Check sheet for the modelled part. Datum: model origin and axes. Units: mm. Round coordinates to 2 decimals unless told otherwise and drop trailing zeros. Write each loop counter-clockwise with the first axis right and the second up, starting at its lowest first coordinate (ties: lowest second). Pieces come first, ordered by that corner, then holes. Notation, with made-up numbers: (60, 74.5) -> (77, 74.5) arc R18 ccw to (77, 79.5) -> close; hole circle Ø4 at (-0.75, 41). An arc over 180 degrees is marked (long way). Answer as a JSON object with one key per item and string values. Group by question number.
```python
from build123d import *

# Parameters (mm, degrees)
BOSS_EXTRUDE12_DEPTH       = 1
SKETCH88_W                 = 60
SKETCH88_H                 = 110
CUT_EXTRUDE1_DEPTH         = 1
FILLET1_R                  = 10
M2_5_CLEARANCE_HOLE1_D     = 2.9
M2_5_CLEARANCE_HOLE1_DEPTH = 11.5
SKETCH91_W                 = 8
SKETCH91_H                 = 15
SKETCH91_R                 = 1.55
BOSS_EXTRUDE13_DEPTH       = 1
FILLET2_R                  = 2
CHAMFER1_SIZE              = 1.5
SKETCH93_R                 = 1.25
CUT_EXTRUDE2_DEPTH         = 10
M2_5_CLEARANCE_HOLE2_D     = 2.9
M2_5_CLEARANCE_HOLE2_DEPTH = 30


with BuildPart() as part:
    # Sketch87 → Boss-Extrude12 (new body)
    with BuildSketch(Plane.XY):
        Polygon((-40, 70), (-40, -70), (-30, -70), (-30, -60), (30, -60), (30, -70), (40, -70), (40, 70), align=None)
    extrude(amount=BOSS_EXTRUDE12_DEPTH)

    # Sketch88 → Cut-Extrude1 (cut)
    with BuildSketch(Plane.XY.offset(1)):
        with Locations((0, 5)):
            Rectangle(SKETCH88_W, SKETCH88_H)
    extrude(amount=-CUT_EXTRUDE1_DEPTH, mode=Mode.SUBTRACT)

    # Fillet1
    fillet1_edges = [part.edges().sort_by_distance(p)[0] for p in [
        (-30, -50, 0.5),
        (-30, 60, 0.5),
        (30, 60, 0.5),
        (30, -50, 0.5),
    ]]
    fillet(fillet1_edges, radius=FILLET1_R)

    # M2.5 Clearance Hole1
    with Locations(Plane(origin=(0, 0, 0), x_dir=(-1, 0, 0), z_dir=(0, 0, -1))):
        with Locations((35, -65), (35, -55), (-35, -55), (-35, -65), (12, -55), (-12, -55), (-12, 65), (12, 65), (-35, 65), (35, 65), (-35, 55), (35, 55)):
            Hole(M2_5_CLEARANCE_HOLE1_D / 2, depth=M2_5_CLEARANCE_HOLE1_DEPTH)

    # Sketch91 → Boss-Extrude13 (add)
    with BuildSketch(Plane(origin=(0, 0, 0), x_dir=(-1, 0, 0), z_dir=(0, 0, -1))):
        with Locations((-9, -67.5)):
            Rectangle(SKETCH91_W, SKETCH91_H)
        with Locations((-9, -70.5)):
            Circle(SKETCH91_R, mode=Mode.SUBTRACT)
    extrude(amount=-BOSS_EXTRUDE13_DEPTH)

    # Fillet2
    fillet2_edges = [part.edges().sort_by_distance(p)[0] for p in [
        (30, -60, 0.5),
        (-30, -60, 0.5),
        (13, -60, 0.5),
    ]]
    fillet(fillet2_edges, radius=FILLET2_R)

    # Chamfer1
    chamfer1_edges = [part.edges().sort_by_distance(p)[0] for p in [
        (40, 70, 0.5),
        (40, -70, 0.5),
        (-40, -70, 0.5),
        (-40, 70, 0.5),
    ]]
    chamfer(chamfer1_edges, length=CHAMFER1_SIZE)

    # Sketch93 → Cut-Extrude2 (cut)
    with BuildSketch(Plane(origin=(0, 0, 0), x_dir=(-1, 0, 0), z_dir=(0, 0, -1))):
        with Locations((-4.292893219, -60.707106781)):
            Circle(SKETCH93_R)
    extrude(amount=-CUT_EXTRUDE2_DEPTH, mode=Mode.SUBTRACT)

    # M2.5 Clearance Hole2
    with Locations(Plane(origin=(0, 0, 0), x_dir=(-1, 0, 0), z_dir=(0, 0, -1))):
        with Locations((-36, 14), (-36, -6)):
            m2_5_clearance_hole2 = Hole(M2_5_CLEARANCE_HOLE2_D / 2, depth=M2_5_CLEARANCE_HOLE2_DEPTH)

    # Mirror1: M2.5 Clearance Hole2 across plane
    add(m2_5_clearance_hole2.mirror(Plane(origin=(0, 0, 0), x_dir=(0, 0, 1), z_dir=(1, 0, 0))), mode=Mode.SUBTRACT)


solid = part.part
```
(1) Scan lines: line 1 along Y through (x, z) = (9, 0.3); line 2 along X through (y, z) = (-65, 0.35); line 3 along X through (y, z) = (65, 0.65). Record each from-to range of solid material in increasing order.
(2) Section check C-C on x = -12. Record the cut outline in (y, z), then the cut area to 3 significant figures.
(3) Go/stop test with flat-tipped pins: pin 1 Ø2.5 at (x, y) = (-12, -55) entering from +Z; pin 2 Ø3.5 at (x, y) = (12, 65) entering from -Z. Record where each tip stops, or that it passes through.
(4) Section check A-A on x = 9. Record the cut outline in (y, z), then the cut area to 3 significant figures.
(5) Section check D-D on x = -23.5. Record the cut outline in (y, z), then the cut area to 3 significant figures.
(6) Release check for a two-part mould opening along Y. For faces 1 (the flat face through (-33, 3, 0)), 2 (the cylindrical face through (-34.85, -6.88, 0.51)), 3 (the cylindrical face through (-26.99, -47.15, 0.49)) record: pulls with the +Y half, pulls with the -Y half, needs draft (parallel to the pull), parting line crosses it, or undercut.
(7) Section check B-B on y = -11. Record the cut outline in (x, z).
Data:
{
 "1": {"line 1": "y = -75 to -72.05, -68.95 to -50, 60 to 70", "line 2": "x = -40 to -36.45, -33.55 to -30, 5 to 13, 30 to 33.55, 36.45 to 40", "line 3": "x = -40 to -36.45, -33.55 to -13.45, -10.55 to 10.55, 13.45 to 33.55, 36.45 to 40"},
 "2": {"outline": "(-60, 0) -> (-56.45, 0) -> (-56.45, 1) -> (-60, 1) -> close; (-53.55, 0) -> (-50, 0) -> (-50, 1) -> (-53.55, 1) -> close; (60, 0) -> (63.55, 0) -> (63.55, 1) -> (60, 1) -> close; (66.45, 0) -> (70, 0) -> (70, 1) -> (66.45, 1) -> close", "area": "14.2 mm²"},
 "3": {"pin 1": "passes through", "pin 2": "stops at z = 0"},
 "4": {"outline": "(-75, 0) -> (-72.05, 0) -> (-72.05, 1) -> (-75, 1) -> close; (-68.95, 0) -> (-50, 0) -> (-50, 1) -> (-68.95, 1) -> close; (60, 0) -> (70, 0) -> (70, 1) -> (60, 1) -> close", "area": "31.9 mm²"},
 "5": {"outline": "(-60, 0) -> (-49.37, 0) -> (-49.37, 1) -> (-60, 1) -> close; (59.37, 0) -> (70, 0) -> (70, 1) -> (59.37, 1) -> close", "area": "21.3 mm²"},
 "6": {"face 1": "needs draft", "face 2": "undercut", "face 3": "undercut"},
 "7": {"outline": "(-40, 0) -> (-30, 0) -> (-30, 1) -> (-40, 1) -> close; (30, 0) -> (40, 0) -> (40, 1) -> (30, 1) -> close"}
}
